Input: part model. Units: mm. Frame: model coordinates. Give positions to 0.01 mm unless a question says otherwise; leave off trailing zeros. Loops run counter-clockwise (first coordinate to the right, second up) from the corner with the lowest first, then second, coordinate; pieces in that order, holes last. Notation, with made-up numbers: (-21.5, -6.75) -> (-5.5, -6.75) arc R25 cw to (-5.5, 32.25) -> close; hole circle Ø8 at (75.25, 70). An arc over 180 degrees is marked (long way). Answer as a JSON object with one key per item and string values.
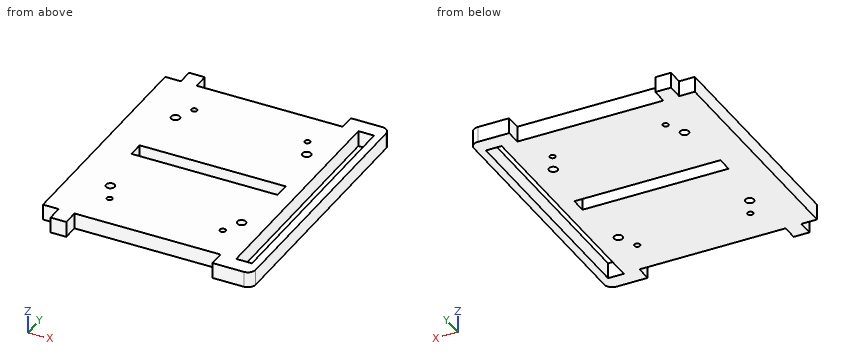
```python
from build123d import *

# Parameters (mm, degrees)
SKETCH1_W                 = 59.0248375
SKETCH1_H                 = 6.35
SKETCH1_W_2               = 6.35
SKETCH1_H_2               = 95.25
BOSS_EXTRUDE1_DEPTH       = 6.35
TAP_DRILL_FOR_8_32_TAP4_D = 3.4544
TAP_DRILL_FOR_8_32_TAP5_D = 3.4544
TAP_DRILL_FOR_4_40_TAP1_D = 2.2606


with BuildPart() as part:
    # Sketch1 → Boss-Extrude1 (new body)
    with BuildSketch(Plane.XY):
        with BuildLine():
            Line((-36.4109, 0), (-30.0609, 0))
            Line((-30.0609, 0), (-30.0609, 6.35))
            Line((-30.0609, 6.35), (28.9639375, 6.35))
            Line((28.9639375, 6.35), (28.9639375, 0))
            Line((28.9639375, 0), (41.6639375, 0))
            ThreePointArc((41.6639375, 0), (43.90900153, 0.92993597), (44.8389375, 3.175))
            Line((44.8389375, 3.175), (44.8389375, 104.775))
            ThreePointArc((44.8389375, 104.775), (43.90900153, 107.02006403), (41.6639375, 107.95))
            Line((41.6639375, 107.95), (28.9639375, 107.95))
            Line((28.9639375, 107.95), (28.9639375, 101.6))
            Line((28.9639375, 101.6), (-30.0609, 101.6))
            Line((-30.0609, 101.6), (-30.0609, 107.95))
            Line((-30.0609, 107.95), (-36.4109, 107.95))
            Line((-36.4109, 107.95), (-36.4109, 101.6))
            Line((-36.4109, 101.6), (-42.7609, 101.6))
            Line((-42.7609, 101.6), (-42.7609, 6.35))
            Line((-42.7609, 6.35), (-36.4109, 6.35))
            Line((-36.4109, 6.35), (-36.4109, 0))
        make_face()
        with Locations((-0.54848125, 53.975)):
            Rectangle(SKETCH1_W, SKETCH1_H, mode=Mode.SUBTRACT)
        with Locations((38.4889375, 53.975)):
            Rectangle(SKETCH1_W_2, SKETCH1_H_2, mode=Mode.SUBTRACT)
    extrude(amount=BOSS_EXTRUDE1_DEPTH)

    # Tap Drill for #8-32 Tap4 (through all)
    with Locations(Plane(origin=(210.206342913, -81.87086846, 83.327875), x_dir=(1, 0, 0), z_dir=(0, 0, 1))):
        with Locations((-184.233255413, 161.24586846), (-184.233255413, 110.44586846), (-237.276392913, 110.44586846), (-237.276392913, 161.24586846)):
            Hole(TAP_DRILL_FOR_8_32_TAP4_D / 2)

    # Tap Drill for #8-32 Tap5 (through all)
    with Locations(Plane(origin=(210.206342913, -81.87086846, 6.35), x_dir=(1, 0, 0), z_dir=(0, 0, 1))):
        with Locations((-184.233255413, 161.24586846), (-184.233255413, 110.44586846), (-237.276392913, 110.44586846), (-237.276392913, 161.24586846)):
            Hole(TAP_DRILL_FOR_8_32_TAP5_D / 2)

    # Tap Drill for #4-40 Tap1 (through all)
    with Locations(Plane(origin=(210.206342913, -81.87086846, 0), x_dir=(-1, 0, 0), z_dir=(0, 0, -1))):
        with Locations((233.614824163, 168.86586846), (233.614824163, 102.82586846), (187.894824163, 102.82586846), (187.894824163, 168.86586846)):
            Hole(TAP_DRILL_FOR_4_40_TAP1_D / 2)


solid = part.part
```
Q1. Section C-C, the plane y = 56. Return the cut outline in (x, z), then the cut area to 3 significant figures.
Evaluation:
{"outline": "(-42.76, 0) -> (-30.06, 0) -> (-30.06, 6.35) -> (-42.76, 6.35) -> close; (28.96, 0) -> (35.31, 0) -> (35.31, 6.35) -> (28.96, 6.35) -> close; (41.66, 0) -> (44.84, 0) -> (44.84, 6.35) -> (41.66, 6.35) -> close", "area": "141 mm2"}
Q2. Section B-B, the plane x = -5. Return the cut outline in (y, z).
Evaluation:
{"outline": "(6.35, 0) -> (50.8, 0) -> (50.8, 6.35) -> (6.35, 6.35) -> close; (57.15, 0) -> (101.6, 0) -> (101.6, 6.35) -> (57.15, 6.35) -> close"}
Q3. Section D-D, the plane z = 1.25. Give the number of separate pieces and of enclosed holes in the cut face, then the cut area to 3 significant figures.
Evaluation:
{"separate pieces": "1", "enclosed holes": "10", "area": "7,590 mm2"}
Q4. Pin query (flat end, axial travel): pin 1 (3 mm diameter, centred on y = 105.5, z = 4.5, fed in from -X); pin 2 (2 mm diameter, centred on x = -27.07, y = 28.58, fed in from +Z); pin 3 (1.9 mm diameter, centred on x = -39, z = 4, fed in from +Y); pin 4 (2 mm diameter, centred on x = -10.5, z = 1.5, fed in from -Y). Return the tip coordinate at first contact, or that it passes through.
Evaluation:
{"pin 1": "stops at x = -36.41", "pin 2": "passes through", "pin 3": "stops at y = 101.6", "pin 4": "stops at y = 6.35"}
Q5. Ray query, line 1 along Y through (x, z) = (-27, 5.5); line 2 along X through (y, z) = (46, 3.5); line 3 along Y through (x, z) = (22.5, 6). Return the intervals inside material, ascending.
Evaluation:
{"line 1": "y = 6.35 to 26.85, 30.3 to 50.8, 57.15 to 77.65, 81.1 to 101.6", "line 2": "x = -42.76 to 35.31, 41.66 to 44.84", "line 3": "y = 6.35 to 19.84, 22.07 to 50.8, 57.15 to 85.88, 88.11 to 101.6"}
Q6. Section A-A, the plane y = 35.5. Return the cut outline in (x, z), then the cut area to 3 significant figures.
Evaluation:
{"outline": "(-42.76, 0) -> (35.31, 0) -> (35.31, 6.35) -> (-42.76, 6.35) -> close; (41.66, 0) -> (44.84, 0) -> (44.84, 6.35) -> (41.66, 6.35) -> close", "area": "516 mm2"}
